Here's how the part is built. I have some questions about the finished solid (model axes, mm). Face numbers are marked on the shaded views. A direction names the side the tool comes from. Round coordinates to 2 decimals unless told otherwise and drop trailing zeros. Order: outer loops, then holes, each group sorted by start corner. A loop starts at its lowest first (then second) coordinate and runs counter-clockwise, first axis right, second up. Notation, with made-up numbers: (73.25, -19.5) - (82.25, -19.5) arc R23 cw to (82.25, 7.5) - close; hole circle Ø6 at (-5.75, -18). An arc over 180 degrees is marked (long way). Answer as a JSON object with one key per item and string values.
```python
from build123d import *

# Parameters (mm, degrees)
F0_W      = 58.878030628
F0_H      = 75.4921324551
F1_DEPTH  = 25.4
F3_DEPTH  = 25.4
F4_DEPTH  = 80.01
F5_W      = 16.8407969177
F5_H      = 39.2584712245
F6_DEPTH  = 29.972
F7_W      = 11.6147371009
F7_H      = 37.7531396225
F8_DEPTH  = 27.178
F10_W     = 35.4502582923
F10_H     = 15.3018832207
F11_DEPTH = 14.986


with BuildPart() as f1:
    # F0 (on Top) → F1 (new body)
    with BuildSketch(Plane.XY):
        with Locations((-1.4573782682, -3.2062288374)):
            Rectangle(F0_W, F0_H)
    extrude(amount=F1_DEPTH)

    # F2 (on face) → F3 (cut)
    with BuildSketch(Plane.XY.offset(25.4)):
        with BuildLine():
            ThreePointArc((-5.4399550781, 34.5398373902), (13.6686067521, 27.7903712145), (27.9816370457, 13.4436087683))
            Line((27.9816370457, 13.4436087683), (27.9816370457, 34.5398373902))
            Line((27.9816370457, 34.5398373902), (-5.4399550781, 34.5398373902))
        make_face()
    extrude(amount=-F3_DEPTH, mode=Mode.SUBTRACT)

    # F4 (add): a face of the model
    f4_faces = [f1.faces().sort_by_distance(p)[0] for p in [
        (-2.600266852, -4.9615268336, 25.4),
    ]]
    extrude(f4_faces, amount=F4_DEPTH)

    # F5 (on face) → F6 (cut)
    with BuildSketch(Plane.YZ.offset(27.9816370457)):
        with Locations((-25.2520013601, 25.8709422778)):
            Rectangle(F5_W, F5_H)
    extrude(amount=-F6_DEPTH, mode=Mode.SUBTRACT)

    # F7 (on face) → F8 (cut)
    with BuildSketch(Plane.YZ.offset(27.9816370457)):
        with Locations((-3.284684848, 27.8146467172)):
            Rectangle(F7_W, F7_H)
    extrude(amount=-F8_DEPTH, mode=Mode.SUBTRACT)

    # F10 (on face) → F11 (cut)
    with BuildSketch(Plane.YZ.offset(27.9816370457)):
        with Locations((-13.1954229437, 64.2097368836)):
            Rectangle(F10_W, F10_H)
    extrude(amount=-F11_DEPTH, mode=Mode.SUBTRACT)


solid = f1.part
```
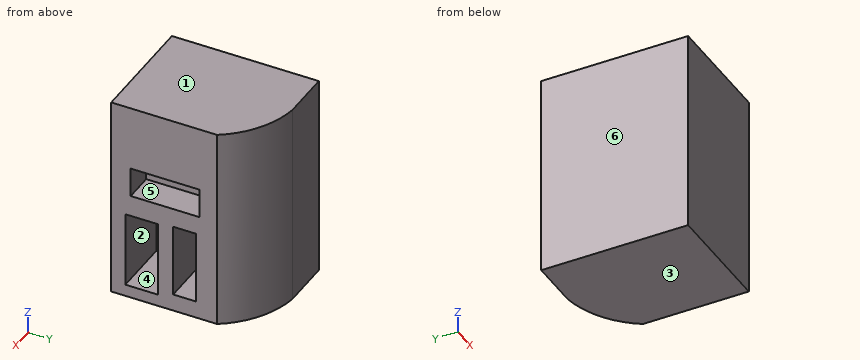
1. Thinking about a two-plate mould opening in Z: for the marked faces 3, 4, 5 and 6, which applies, pulls with the +Z half, pulls with the -Z half, needs draft (parallel to the pull), parting line crosses it, or undercut?
Responses:
{"face 3": "pulls with the -Z half", "face 4": "undercut", "face 5": "undercut", "face 6": "needs draft"}
2. Imagine slicing it at B-B (z = 74.5). List the corners of the cut face in (x, y) for me, plus the area to 3 significant figures.
Responses:
{"outline": "(-30.9, -40.95) - (27.98, -40.95) - (27.98, 13.44) arc R45.71 ccw to (-5.44, 34.54) - (-30.9, 34.54) - close", "area": "4,210 mm2"}
3. If I drill on L1, parallel to Z at x = 2, y = -8; L2, parallel to Y at x = 2, z = 18; L3, parallel to Y at x = 6, z = 14.5, over which ranges is the centre line in solid material (lowest first)? Write a range as [from, to].
Responses:
{"L1": "[0, 8.94], [46.69, 105.41]", "L2": "[-40.95, -33.67], [-16.83, -9.09], [2.52, 33.04]", "L3": "[-40.95, -33.67], [-16.83, -9.09], [2.52, 31.68]"}
4. Imagine slicing it at D-D (x = 22). List the corners of the cut face in (y, z) for me.
Responses:
{"outline": "(-40.95, 0) - (21.05, 0) - (21.05, 105.41) - (-40.95, 105.41) - close; hole (-33.67, 6.24) - (-16.83, 6.24) - (-16.83, 45.5) - (-33.67, 45.5) - close; hole (-30.92, 56.56) - (4.53, 56.56) - (4.53, 71.86) - (-30.92, 71.86) - close; hole (-9.09, 8.94) - (2.52, 8.94) - (2.52, 46.69) - (-9.09, 46.69) - close"}
5. Imagine slicing it at C-C (y = -20.5). List the corners of the cut face in (x, z) for me, plus the area to 3 significant figures.
Responses:
{"outline": "(-30.9, 0) - (27.98, 0) - (27.98, 6.24) - (-1.99, 6.24) - (-1.99, 45.5) - (27.98, 45.5) - (27.98, 56.56) - (13, 56.56) - (13, 71.86) - (27.98, 71.86) - (27.98, 105.41) - (-30.9, 105.41) - close", "area": "4,800 mm2"}
6. For P1, Ø7.5, axis at x = 22, y = -8, coming from the -Z side; P2, Ø4.5, axis at x = 17, z = 66, coming from the +Y side; P3, Ø1, axis at x = 21.5, z = 45.5, coming from the +Y side; P4, Ø7.5, axis at y = -17, z = 61, coming from the +X side, each with a flat end and sliding along its axis, tell me the tip position at first contact or that it passes through.
Responses:
{"P1": "z = 0", "P2": "y = 27.09", "P3": "y = 22.04", "P4": "x = 13"}
7. Imagine slicing it at A-A (x = 9). List the corners of the cut face in (y, z) for me, plus the area to 3 significant figures.
Responses:
{"outline": "(-40.95, 0) - (30.37, 0) - (30.37, 105.41) - (-40.95, 105.41) - close; hole (-33.67, 6.24) - (-16.83, 6.24) - (-16.83, 45.5) - (-33.67, 45.5) - close; hole (-9.09, 8.94) - (2.52, 8.94) - (2.52, 46.69) - (-9.09, 46.69) - close", "area": "6,420 mm2"}
8. For the marked faces 1 and 2, which set-ups out of +Z, -Z, +X, -X, +Y, -Y let a thin tool reach every point of the face, with its end or its side?
Responses:
{"face 1": "+Z, +X, -X, +Y, -Y", "face 2": "+X"}
